Study the drawing (mm; zero at the part's minimum x, y, z) and answer. A direction names the side the tool comes from. Coordinates: 2 decimals unless noted, no trailing zeros. Loops run counter-clockwise (first coordinate to the right, second up) from the corner with the lowest first, then second, coordinate; pieces in that order, holes last. Notation, with made-up numbers: (39, 6.5) -> (98, 6.5) arc R18 ccw to (98, 40.5) -> close; hole circle Ø1 at (16, 17.25). An arc over 180 degrees is marked (long way). Answer in a Markdown table with one row per item.
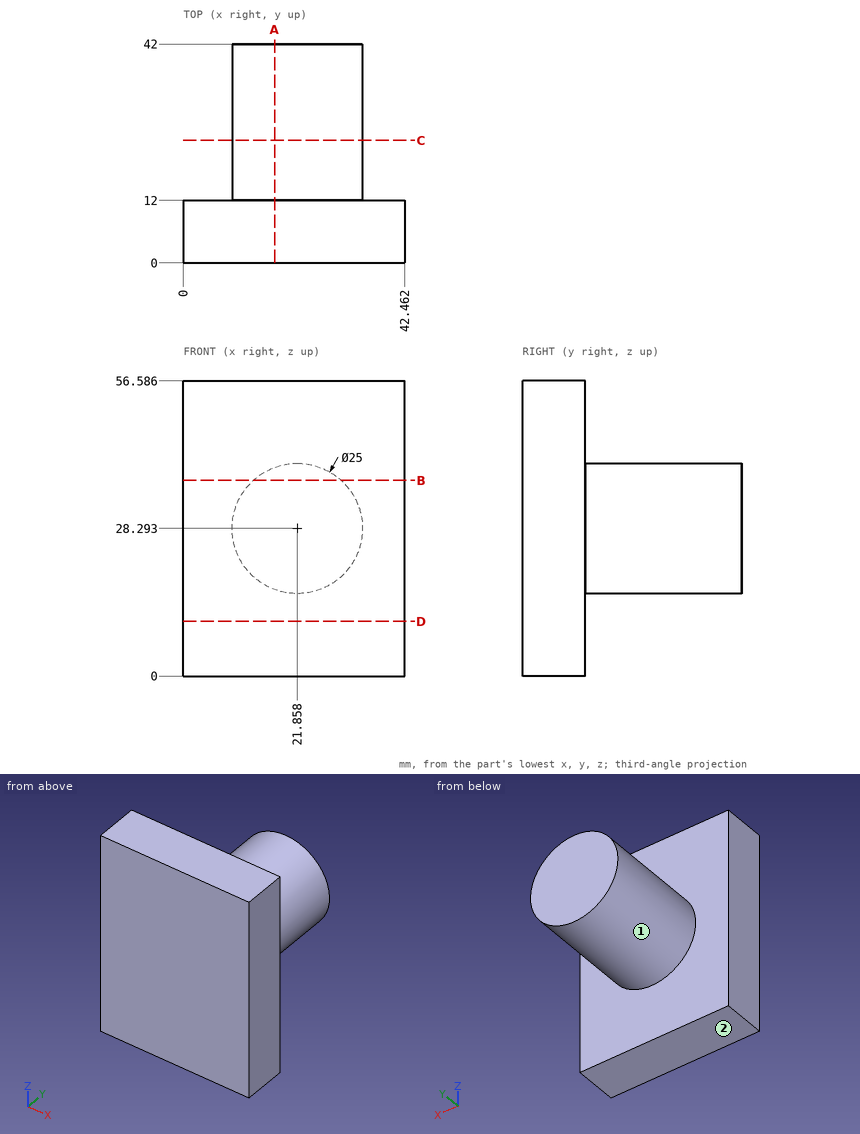
1. A cutting plane is placed at C-C on y = 23.5. Give the vertices of the cut face in (x, z), and give its area (3 significant figures).
A:
| item | result |
|---|---|
| outline | circle Ø25 at (21.86, 28.29) |
| area | 491 mm2 |
2. A cutting plane is placed at A-A on x = 17.5. Give the vertices of the cut face in (y, z), and give its area (3 significant figures).
A:
| item | result |
|---|---|
| outline | (0, 0) -> (12, 0) -> (12, 16.58) -> (42, 16.58) -> (42, 40.01) -> (12, 40.01) -> (12, 56.59) -> (0, 56.59) -> close |
| area | 1,380 mm2 |
3. A cutting plane is placed at B-B on z = 37.5. Give the vertices of the cut face in (x, y), and give its area (3 significant figures).
A:
| item | result |
|---|---|
| outline | (0, 0) -> (42.46, 0) -> (42.46, 12) -> (30.31, 12) -> (30.31, 42) -> (13.4, 42) -> (13.4, 12) -> (0, 12) -> close |
| area | 1,020 mm2 |
4. Given pin 1 Ø2 at (x, y) = (6.5, 32.5) entering from -Z; pin 2 Ø12 at (y, z) = (23, 15.5) entering from -X (1 decimal); pin 3 Ø10 at (y, z) = (30, 32) entering from -X; pin 4 Ø1.5 at (x, y) = (24.5, 37.5) entering from -Z, each flat-ended and moving along its own axis, determine where each tip first touches the part or whether it passes through.
A:
| item | result |
|---|---|
| pin 1 | passes through |
| pin 2 | stops at x = 11.4 |
| pin 3 | stops at x = 9.36 |
| pin 4 | stops at z = 15.94 |
5. A cutting plane is placed at D-D on z = 10.5. Give the vertices of the cut face in (x, y).
A:
| item | result |
|---|---|
| outline | (0, 0) -> (42.46, 0) -> (42.46, 12) -> (0, 12) -> close |
6. A tool of negligible diameter and unlimited length cuts with its end or side. For the marked faces 1 and 2, from which of +Z, -Z, +X, -X, +Y, -Y can it reach the whole face along a straight path? Write none if from no direction.
A:
| item | result |
|---|---|
| face 1 | +Y |
| face 2 | -Z, +X, -X, +Y, -Y |
7. Find the intervals of material crossed by probe 1 along Y at (x, z) = (9, 32.5); probe 2 along Z at (x, y) = (22, 40.5); probe 3 along Z at (x, y) = (23, 34.5) (1 decimal), in increasing order.
A:
| item | result |
|---|---|
| probe 1 | y = 0 to 12 |
| probe 2 | z = 15.79 to 40.79 |
| probe 3 | z = 15.8 to 40.7 |
